The listing builds one solid part. Answer for the finished solid, in the listing's coordinates (mm). Face numbers are marked on the shaded views. A direction names the side the tool comes from. Give positions to 0.01 mm unless a question says otherwise; leave off trailing zeros. Order: outer loops, then holes, each group sorted by start corner. A loop starts at its lowest first (then second) coordinate and runs counter-clockwise, first axis right, second up. Notation, with made-up numbers: (9.25, -37) - (24.25, -37) arc R21 cw to (24.25, -28) - close; hole circle Ø2 at (50.25, -26.75). An arc over 180 degrees is marked (long way). Use a Markdown table: item, result. Add a question column.
1) Find section B-B, the plane y = 0. Determine the outline of the cut face in (x, z) (3 decimals).
2) Straight lines are drawn through the part: line 1 (Z direction, x = 7.5, y = 12.25); line 2 (Z direction, x = -12, y = 0.25); line 3 (Z direction, x = 1, y = 9.25). For each, find the intervals that lie inside material, in ascending order.
3) Flat-ended cylindrical pins translate along their axes: pin 1 (6.5 mm diameter, centred on x = 1.5, z = 20.5, fed in from +Y); pin 2 (6 mm diameter, centred on y = 2, z = 20.5, fed in from -X); pin 3 (3 mm diameter, centred on x = 11, z = 107, fed in from -Y). Find the tip coordinate at first contact, or state that the pin passes through.
4) Find section C-C, the plane z = 45. Determine the outline of the cut face in (x, y).
5) For the marked faces 1, 2 and 3, determine the directions among +Z, -Z, +X, -X, +Y, -Y from which every point of the face is accessible in a straight line to the end or side of a thin tool.
6) Find section D-D, the plane x = 12. Determine the outline of the cut face in (y, z), plus the area to 3 significant figures.
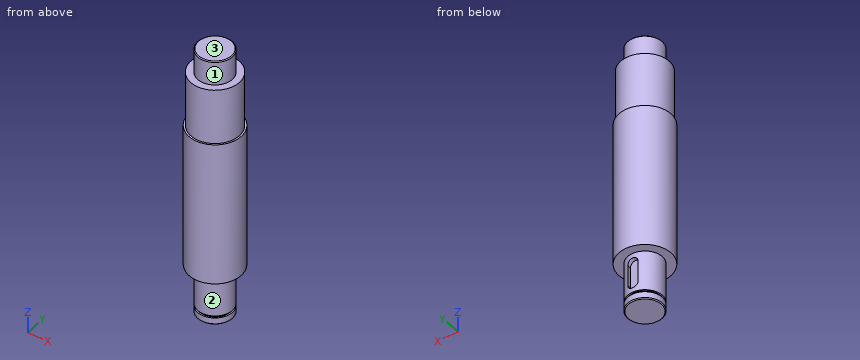
Autodesk Inventor part; units mm, degrees
ref_plane "工作平面1" through (0, 10, 0) normal (0, 1, 0) x (-1, 0, 0)
ref_plane "YZ Plane" through (0, 0, 0) normal (1, 0, 0) x (0, 1, 0)
ref_plane "XY Plane" through (0, 0, 0) normal (0, 0, 1) x (1, 0, 0)
sketch "草图1" plane through (0, 0, 0) normal (0, 0, 1) x (1, 0, 0)
  circle A0 centre (0, 0) radius 10
  dimension "d0" = 20
extrude "拉伸1" add sketch "草图1" along normal blind 28.378
sketch "草图2" plane through (0, 0, 28.378) normal (0, 0, 1) x (1, 0, 0)
  circle A0 centre (0, 0) radius 15
  dimension "d3" = 30
extrude "拉伸2" add sketch "草图2" along normal blind 83.422
sketch "草图3" plane through (0, 0, 111.8) normal (0, 0, 1) x (1, 0, 0)
  circle A0 centre (0, 0) radius 14
  dimension "d6" = 28
extrude "拉伸3" add sketch "草图3" along normal blind 32
sketch "草图4" plane through (0, 0, 143.8) normal (0, 0, 1) x (1, 0, 0)
  circle A0 centre (0, 0) radius 10
  dimension "d9" = 20
extrude "拉伸4" add sketch "草图4" along normal blind 14
ref_plane "工作平面1" through (0, 10, 0) normal (0, 1, 0) x (-1, 0, 0)
sketch "草图5" plane through (0, 10, 0) normal (0, 1, 0) x (-1, 0, 0)
  line L0 (-3, 22.789) -> (3, 22.789)
  line L1 (3, 22.789) -> (3, 10.789)
  line L2 (3, 10.789) -> (-3, 10.789)
  line L3 (-3, 10.789) -> (-3, 22.789)
  arc A0 (3, 22.789) -> (-3, 22.789) centre (0, 22.789) ccw
  arc A1 (-3, 10.789) -> (3, 10.789) centre (0, 10.789) ccw
  line L4 (0, 0) -> (0, -4.7288)
  line L5 (10, 28.378) -> (-10, 28.378)
  dimension "d12" = 4.7288
  dimension "d13" = 6
  dimension "d14" = 12
  dimension "d21" = 5.589
extrude "拉伸5" cut sketch "草图5" against normal blind 2.5
chamfer "倒角1" distance 0.5 angle 45 2 edges at (-10, 0, 0) (-10, 0, 157.8)
sketch "草图6" plane through (0, 0, 0) normal (0, 1, 0) x (-1, 0, 0)
  line L0 (14.4109, 5.2) -> (9.175, 5.2)
  line L1 (9.175, 5.2) -> (9.175, 4)
  line L2 (9.175, 4) -> (14.4109, 4)
  line L3 (14.4109, 4) -> (14.4109, 5.2)
  line L4 (9.5, 0) -> (-9.5, 0)
  line L5 (0, 0) -> (0, -3.7924)
  dimension "d22" = 4
  dimension "d23" = 1.2
  dimension "d24" = 3.7924
  dimension "d25" = 9.175
  dimension "d26" = 5.2359
revolve "旋转1" cut sketch "草图6" angle 360 about axis through (0, 0, 0) along (0, 0, -1)
properties part number "齿轮150配件"
The answers:
| question | item | result |
|---|---|---|
| 1 | outline | (-15, 28.378) - (-10, 28.378) - (-10, 5.2) - (-9.175, 5.2) - (-9.175, 4) - (-10, 4) - (-10, 0.5) - (-9.5, 0) - (9.5, 0) - (10, 0.5) - (10, 4) - (9.175, 4) - (9.175, 5.2) - (10, 5.2) - (10, 28.378) - (15, 28.378) - (15, 111.8) - (14, 111.8) - (14, 143.8) - (10, 143.8) - (10, 157.3) - (9.5, 157.8) - (-9.5, 157.8) - (-10, 157.3) - (-10, 143.8) - (-14, 143.8) - (-14, 111.8) - (-15, 111.8) - close |
| 2 | line 1 | 28.38 to 111.8 |
| 2 | line 2 | 28.38 to 143.8 |
| 2 | line 3 | 0 to 4, 5.2 to 7.96, 25.62 to 157.8 |
| 3 | pin 1 | y = 9.56 |
| 3 | pin 2 | x = -10 |
| 3 | pin 3 | y = -11.61 |
| 4 | outline | circle Ø30 at (0, 0) |
| 5 | face 1 | +Z |
| 5 | face 2 | -Z |
| 5 | face 3 | +Z, +X, -X, +Y, -Y |
| 6 | outline | (-9, 28.38) - (9, 28.38) - (9, 111.8) - (7.21, 111.8) - (7.21, 143.8) - (-7.21, 143.8) - (-7.21, 111.8) - (-9, 111.8) - close |
| 6 | area | 1,960 mm2 |
